Autodesk Inventor part; units mm, degrees
ref_plane "YZ Plane" through (0, 0, 0) normal (1, 0, 0) x (0, 1, 0)
ref_plane "XZ Plane" through (0, 0, 0) normal (0, 1, 0) x (-1, 0, 0)
ref_plane "XY Plane" through (0, 0, 0) normal (0, 0, 1) x (1, 0, 0)
sketch "スケッチ6" plane through (0, 0, 0) normal (0, 0, 1) x (1, 0, 0)
  line L0 (0, 0) -> (25, 0)
  line L1 (25, 0) -> (25, 30)
  line L2 (25, 30) -> (0, 30)
  line L3 (0, 30) -> (0, 0)
  circle A0 centre (5, 5) radius 2.5
  circle A1 centre (20, 5) radius 2.5
  dimension "d39" = 5
  dimension "d40" = 5
  dimension "d41" = 5
  dimension "d42" = 5
  dimension "d43" = 15
  dimension "d44" = 5
  dimension "d45" = 5
  dimension "d46" = 30
extrude "押し出し4" add sketch "スケッチ6" along normal blind 5
sketch "スケッチ7" plane through (0, 0, 5) normal (0, 0, 1) x (1, 0, 0)
  line L0 (25, 30) -> (0, 30)
  line L1 (10, 30) -> (15, 30)
  line L2 (15, 30) -> (15, 10)
  line L3 (15, 10) -> (10, 10)
  line L4 (10, 10) -> (10, 30)
  line L5 (25, 0) -> (25, 30)
  line L6 (0, 30) -> (0, 0)
  line L7 (0, 0) -> (25, 0)
  line L8 (10, 30) -> (15, 30)
  line L9 (15, 30) -> (15, 35)
  line L10 (15, 35) -> (10, 35)
  line L11 (10, 35) -> (10, 30)
  dimension "d49" = 5
  dimension "d50" = 10
  dimension "d51" = 10
  dimension "d52" = 10
  dimension "d55" = 5
  dimension "d56" = 5
extrude "押し出し5" add sketch "スケッチ7" along normal blind 10 contours L2 L3 L4 L0 | L0 L11 L10 L9
sketch "スケッチ8" plane through (10, 30, 5) normal (-1, 0, 0) x (0, 0, 1)
  line L0 (10, 5) -> (10, -20)
  line L1 (0, 5) -> (10, 5)
  line L2 (0, -20) -> (10, -20)
  point P0 (-5, -30)
  point P1 (3.1, -13.5)
  point P2 (3.1, -1.5)
  dimension "d57" = 6.9
  dimension "d58" = 6.9
  dimension "d59" = 12
  dimension "d60" = 6.5
  dimension "d61" = 6.5
hole "穴3" at (10, 16.5, 8.1) at (10, 28.5, 8.1) direction (1, 0, 0) diameter 5 depth 8
sketch "スケッチ9" plane through (0, 0, 5) normal (0, 0, 1) x (1, 0, 0)
  line L0 (10, 30) -> (0, 30)
  line L1 (0, 30) -> (7, 30)
  line L2 (7, 30) -> (7, 10)
  line L3 (7, 10) -> (0, 10)
  line L4 (0, 10) -> (0, 30)
  line L5 (25, 0) -> (25, 30)
  line L6 (25, 30) -> (18, 30)
  line L7 (18, 30) -> (18, 10)
  line L8 (18, 10) -> (25, 10)
  line L9 (25, 10) -> (25, 30)
  point P0 (0, 0)
  point P1 (5, 30)
  point P2 (18, 20)
  point P3 (7, 20)
  dimension "d70" = 20
  dimension "d72" = 7
  dimension "d73" = 7
extrude "押し出し6" cut sketch "スケッチ9" against normal blind 10
sketch "スケッチ10" plane through (0, 0, 5) normal (0, 0, 1) x (1, 0, 0)
  line L0 (10, 30) -> (7, 30)
  line L1 (7, 30) -> (7, 10)
  line L2 (7, 10) -> (0, 10)
  line L3 (0, 10) -> (0, 0)
  line L4 (0, 0) -> (25, 0)
  line L5 (25, 0) -> (25, 10)
  line L6 (25, 10) -> (18, 10)
  line L7 (18, 10) -> (18, 30)
  line L8 (18, 30) -> (15, 30)
  circle A0 centre (5, 5) radius 2.5
  circle A1 centre (20, 5) radius 2.5
  line L9 (2, 8) -> (23, 8)
  line L10 (23, 8) -> (23, 2)
  line L11 (23, 2) -> (2, 2)
  line L12 (2, 2) -> (2, 8)
  line L13 (2, 10) -> (2, 0)
  line L14 (24, 10) -> (19, 10)
  line L15 (23, 10) -> (23, 0)
  line L16 (15, 30) -> (15, 10)
  line L17 (15, 10) -> (10, 10)
  line L18 (10, 10) -> (10, 30)
  point P0 (2, 2)
  point P1 (23, 2)
  dimension "d77" = 2
  dimension "d78" = 2
  dimension "d79" = 2
  dimension "d80" = 2
extrude "押し出し7" cut sketch "スケッチ10" against normal blind 4 contours L18 L17 L16 L8 L7 L6 L15 L9 L13 L2 L1 L0 | L13 L12 L4 L3 L2 | L9 L10 L11 L12 | L15 L6 L5 L4 L10 | L11 L15 L4 L13 | A0 | A1
sketch "スケッチ11" plane through (0, 0, 1) normal (0, 0, 1) x (1, 0, 0)
  line L0 (0, 10) -> (0, 0)
  line L1 (25, 0) -> (25, 10)
  line L2 (0, 10) -> (25, 10)
  line L3 (25, 10) -> (25, 0)
  line L4 (25, 0) -> (0, 0)
  line L5 (0, 0) -> (0, 10)
extrude "押し出し8" add sketch "スケッチ11" along normal blind 4
sketch "スケッチ12" plane through (0, 0, 5) normal (0, 0, 1) x (1, 0, 0)
  circle A0 centre (5, 5) radius 2.5
  circle A1 centre (20, 5) radius 2.5
  point P0 (0, 0)
hole "穴4" at (5, 5, 5) at (20, 5, 5) direction (0, 0, -1) diameter 5 depth 8
sketch "スケッチ13" plane through (10, 30, 5) normal (-1, 0, 0) x (0, 0, 1)
  line L0 (10, -20) -> (10, 5)
  line L1 (0, -20) -> (10, -20)
  line L2 (10, 5) -> (7, 5)
  line L3 (7, 5) -> (7, -20)
  line L4 (7, -20) -> (10, -20)
  line L5 (10, -20) -> (10, 5)
  line L6 (-4, 0) -> (-4, -20)
  line L7 (-4, -20) -> (-1, -20)
  line L8 (-1, -20) -> (-1, 5)
  line L9 (-1, 5) -> (-4, 5)
  line L10 (-4, 5) -> (-4, -20)
  point P0 (-5, -30)
  dimension "d93" = 3
  dimension "d94" = 3
extrude "押し出し9" cut sketch "スケッチ13" against normal through all contours L1 L3 L2 L0
sketch "スケッチ14" plane through (10, 30, 5) normal (0, 1, 0) x (1, 0, 0)
  line L0 (5, 4) -> (8, 4)
  line L1 (8, 4) -> (8, 5)
  line L2 (8, 5) -> (-3, 5)
  line L3 (-3, 5) -> (-3, 4)
  line L4 (-3, 4) -> (0, 4)
  line L5 (0, 4) -> (0, 0)
  line L6 (5, 0) -> (0, 0)
  line L7 (5, 0) -> (5, 4)
  point P0 (-10, 5)
extrude "押し出し10" add sketch "スケッチ14" along normal blind 5
sketch "スケッチ15" plane through (0, 0, 1) normal (0, 0, 1) x (1, 0, 0)
  line L0 (7, 10) -> (10, 10)
  line L1 (10, 35) -> (10, 10)
  line L2 (7, 35) -> (10, 35)
  line L3 (7, 10) -> (7, 35)
  line L4 (15, 10) -> (18, 10)
  line L5 (18, 35) -> (18, 10)
  line L6 (15, 35) -> (18, 35)
  line L7 (15, 10) -> (15, 35)
  point P0 (0, 0)
extrude "押し出し11" add sketch "スケッチ15" along normal blind 3
sketch "スケッチ16" plane through (0, 0, 5) normal (0, 0, 1) x (1, 0, 0)
  line L0 (25, 0) -> (25, 10)
  line L1 (10, 10) -> (0, 10)
  line L2 (25, 10) -> (15, 10)
  line L3 (10, 10) -> (15, 10)
  line L4 (0, 10) -> (0, 0)
  line L5 (0, 0) -> (25, 0)
  circle A0 centre (20, 5) radius 2.5
  circle A1 centre (5, 5) radius 2.5
  line L6 (2, 10) -> (2, 0)
  line L7 (23, 10) -> (23, 0)
  point P0 (23, 0)
  point P1 (2, 0)
extrude "押し出し12" cut sketch "スケッチ16" against normal blind 3 contours L5 L7 L2 L0 | L5 L4 L1 L6
fillet "フィレット7" radius 2 4 edges at (2, 10, 3.5) (2, 0, 3.5) (23, 10, 3.5) (23, 0, 3.5)
sketch "スケッチ17" plane through (0, 0, 4) normal (0, 0, 1) x (1, 0, 0)
  line L0 (10, 35) -> (10, 10)
  line L1 (10, 35) -> (7, 35)
  line L2 (7, 35) -> (7, 10)
  line L3 (18, 10) -> (18, 35)
  line L4 (18, 35) -> (15, 35)
  line L5 (15, 10) -> (15, 35)
  line L6 (18, 10) -> (15, 10)
  line L7 (10, 10) -> (7, 10)
  point P0 (0, 0)
extrude "押し出し13" cut sketch "スケッチ17" against normal through all
sketch "スケッチ18" plane through (0, 0, 5) normal (0, 0, 1) x (1, 0, 0)
  line L0 (10, 10) -> (4, 10)
  line L1 (10, 10) -> (7, 10)
  line L2 (7, 10) -> (7, 7)
  line L3 (7, 7) -> (10, 7)
  line L4 (10, 7) -> (10, 10)
  line L5 (21, 10) -> (15, 10)
  line L6 (15, 10) -> (18, 10)
  line L7 (18, 10) -> (18, 7)
  line L8 (18, 7) -> (15, 7)
  line L9 (15, 7) -> (15, 10)
  point P0 (0, 0)
  dimension "d107" = 3
  dimension "d108" = 3
  dimension "d109" = 3
extrude "押し出し14" cut sketch "スケッチ18" against normal blind 10
fillet "フィレット8" radius 0.2 6 edges at (7, 10, 2.5) (7, 7, 2.5) (18, 10, 2.5) (15, 7, 2.5) (10, 7, 2.5) (18, 7, 2.5)
fillet "フィレット9" radius 2 7 edges at (0, 10, 1) (0, 0, 1) (12.5, 35, 12) (12.5, 10, 12) (12.5, 10, 5) (25, 10, 1) (25, 0, 1)
equation "\"d42\" = d41"
equation "\"d45\" = d44"
equation "\"d73\" = d72"
equation "\"d94\" = d93"
equation "\"d108\" = d107"
properties part number "BP_BOX-Support-Bar-Connect1-20" material "ABS プラスチック"
The listing builds one solid part. Answer for the finished solid, in the listing's coordinates (mm). A direction names the side the tool comes from. Coordinates: 2 decimals unless noted, no trailing zeros. Loops run counter-clockwise (first coordinate to the right, second up) from the corner with the lowest first, then second, coordinate; pieces in that order, holes last. Notation, with made-up numbers: M -17.75,87.25 L 18.25,87.25 A31 cw 18.25,120.25 Z; hole C 53.25,23.25 d4. An arc over 180 degrees is marked long. Answer as CSV lines item,"result". Start each with the question number.
(1) For faces 1 (the cylindrical face through (2.57, 9.4, 3.48)), 2 (the cylindrical face through (22.43, 0.6, 3.48)), 3 (the flat face through (18, 9, 3)), 4 (the flat face through (23, 5, 4)), 5 (the cylindrical face through (2.6, 0.57, 3.48)), determine the directions among +Z, -Z, +X, -X, +Y, -Y from which every point of the face is accessible in a straight line to the end or side of a thin tool.
(2) The part is cut by section D-D (y = 5). Give the vertices of the cut face in (x, z), and give its area (3 significant figures).
(3) The part is cut by section A-A (y = 28.5). Give the vertices of the cut face in (x, z), and give its area (3 significant figures).
(4) The mould has two halves that part along X. Classify faces 6 (the cylindrical face through (24.4, 9.43, 0.99)), 7 (the flat face through (8, 7, 3)), 8 (the flat face through (13, 10, 9)), 9 (the flat face through (7, 9, 3)): pulls with the +X half, pulls with the -X half, needs draft (parallel to the pull), parting line crosses it, or undercut.
(5) Given pin 1 (8 mm diameter, centred on x = 9.5, y = 6.5, fed in from +Z); pin 2 (1.2 mm diameter, centred on x = 22.5, y = 3.5, fed in from +Z); pin 3 (0.8 mm diameter, centred on y = 8, z = 3, fed in from +X), each flat-ended and moving along its own axis, determine where each tip first touches the part or whether it passes through.
(6) The part is cut by section C-C (z = 3.5). Give the vertices of the cut face in (x, y), and give its area (3 significant figures).
(7) The part is cut by section B-B (x = 20). Give the vertices of the cut face in (y, z), and give its area (3 significant figures).
(8) Find the intervals of material crossed by L1, parallel to Y at x = 13.8, z = 8.1; L2, parallel to X at y = 5, z = 1.85; L3, parallel to X at y = 5, z = 2.9, in increasing order. Write a range as [from, to].
Determined:
1,face 1,"+Z, -X, +Y"
1,face 2,"+Z, +X, -Y"
1,face 3,"+Z, -Z, +Y"
1,face 4,"+Z, +X, +Y, -Y"
1,face 5,"+Z, -X, -Y"
2,outline,"M 0,0 L 2.5,0 L 2.5,5 L 2,5 L 2,2 L 0,2 Z; M 7.5,0 L 17.5,0 L 17.5,5 L 7.5,5 Z; M 22.5,0 L 25,0 L 25,2 L 23,2 L 23,5 L 22.5,5 Z"
2,area,"63.0 mm2"
3,outline,"M 10,0 L 15,0 L 15,5.6 L 10,5.6 Z; M 10,10.6 L 15,10.6 L 15,12 L 10,12 Z"
3,area,"35.0 mm2"
4,face 6,"pulls with the +X half"
4,face 7,"undercut"
4,face 8,"needs draft"
4,face 9,"undercut"
5,pin 1,"z = 11.29"
5,pin 2,"z = 5"
5,pin 3,"x = 23"
6,outline,"M 2,2 A2 ccw 4,0 L 21,0 A2 ccw 23,2 L 23,8 A2 ccw 21,10 L 18.2,10 A0.2 ccw 18,9.8 L 18,7.2 A0.2 cw 17.8,7 L 15.2,7 A0.2 cw 15,7.2 L 15,35 L 10,35 L 10,7.2 A0.2 cw 9.8,7 L 7.2,7 A0.2 cw 7,7.2 L 7,9.8 A0.2 ccw 6.8,10 L 4,10 A2 ccw 2,8 Z; hole C 5,5 d5; hole C 20,5 d5"
6,area,"274 mm2"
7,outline,"M 0,0 L 2.5,0 L 2.5,5 L 0,5 Z; M 7.5,0 L 10,0 L 10,5 L 7.5,5 Z"
7,area,"25.0 mm2"
8,L1,"[10, 14], [19, 26], [31, 35]"
8,L2,"[0, 2.5], [7.5, 17.5], [22.5, 25]"
8,L3,"[2, 2.5], [7.5, 17.5], [22.5, 23]"
